Answer from the drawing. Dimensions are ordinates in mm from the lowest x, y and z of the part. A direction names the side the tool comes from. Give positions to 0.01 mm unless a question says otherwise; leave off trailing zeros. Loops run counter-clockwise (first coordinate to the right, second up) from the corner with the lowest first, then second, coordinate; pieces in that order, holes last. Notation, with made-up numbers: (-9, 24) -> (30, 24) arc R21 ccw to (30, 35) -> close; hole circle Ø5 at (-37.5, 32). An arc over 180 degrees is marked (long way). Write each question's results on one line, items separated by ' | '. Start each with the question number.
Item 1: Section D-D on x = 81.5 is taken. State how many separate pieces and enclosed holes the cut face has, and give its area (3 significant figures).
Item 2: Section B-B on z = 14 is taken. Write down the section's boundary in (x, y) (1 decimal).
Item 3: Which of the six approach directions +Z, -Z, +X, -X, +Y, -Y give full straight-line access (tool end or side, diameter ignored) to the marked faces 1 and 2?
Item 4: Section C-C on y = 67.5 is taken. Write down the section's boundary in (x, z) (1 decimal).
Item 5: Each of these flat-tipped pins is pushed along its axis until it touches: P1, Ø4, axis at x = 113, z = 37.5, coming from the -Y side; P2, Ø3, axis at y = 17.5, z = 14, coming from the +X side; P3, Ø23, axis at x = 41.5, z = 7, coming from the +Y side (1 decimal); P4, Ø3, axis at x = 60, y = 22, coming from the +Z side. Where does it stop, or does it pass through?
Item 6: Determine the mould class of the marked faces 3, 4 and 5 for opening direction X: +X half, -X half, draft (parallel to the pull), parting line (faces both ways), or undercut.
Item 7: Find the intervals of material crossed by line 1 (X direction, y = 70, z = 30) (1 decimal); line 2 (Y direction, x = 97, z = 38); line 3 (X direction, y = 51, z = 28), in increasing order.
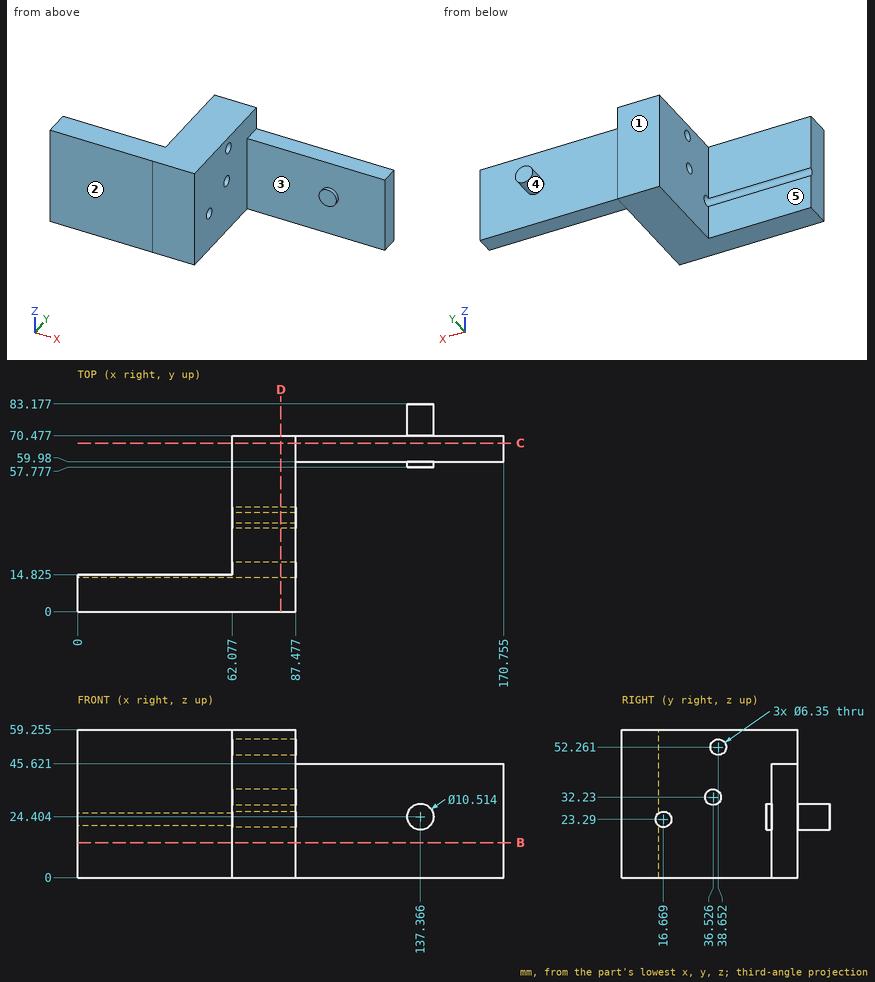
Findings:
1) separate pieces: 1 | enclosed holes: 3 | area: 4,080 mm2
2) outline: (0, 0) -> (87.5, 0) -> (87.5, 60) -> (170.8, 60) -> (170.8, 70.5) -> (62.1, 70.5) -> (62.1, 14.8) -> (0, 14.8) -> close
3) face 1: +Z, -Z, -X, +Y | face 2: +Z, -Z, +X, -X, -Y
4) outline: (62.1, 0) -> (170.8, 0) -> (170.8, 45.6) -> (87.5, 45.6) -> (87.5, 59.3) -> (62.1, 59.3) -> close
5) P1: y = 59.98 | P2: x = 87.48 | P3: y = 14.8 | P4: through
6) face 3: undercut | face 4: parting line | face 5: draft
7) line 1: 62.1 to 170.8 | line 2: 59.98 to 70.48 | line 3: 62.08 to 87.48
